Here's the drawing with two shaded views (mm, measured from the low corner). I have some questions. Coordinates: 2 decimals unless noted, no trailing zeros. Write each loop counter-clockwise with the first axis right and the second up, starting at its lowest first coordinate (ties: lowest second). Pieces come first, ordered by that corner, then holes. Notation, with made-up numbers: (68, -28) -> (106, -28) arc R9 cw to (106, -16) -> close; hole circle Ø8 at (62.25, 76). An arc over 180 degrees is marked (long way). Use one line per item in the form item = value.
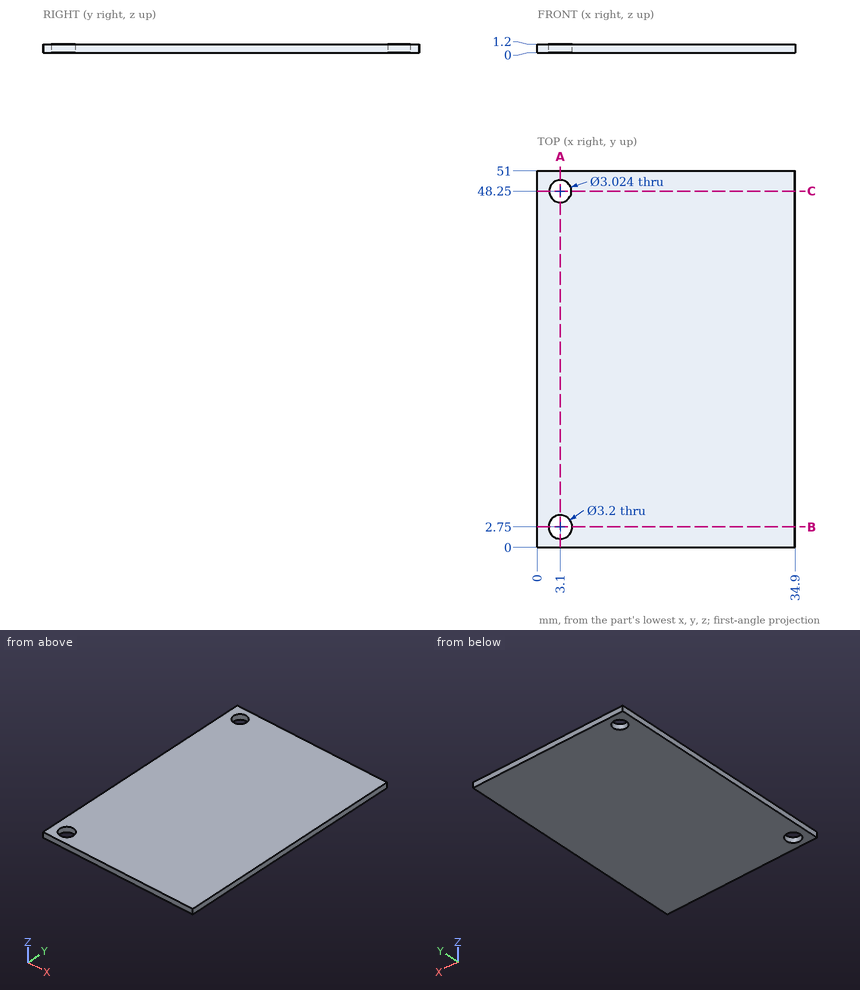
Q1. If I drill on line 1 (Y direction, x = 3.1, z = 0.35); line 2 (Y direction, x = 4, z = 0.5) (1 decimal), over which ranges is the centre line in solid material (lowest first)? Write a range as from..to.
Return value:
line_1 = 0..1.15, 4.35..46.74, 49.76..51
line_2 = 0..1.4, 4.1..47, 49.5..51
Q2. Will this pin go through, and if not, where does the flat tip stop? pin 1 (3 mm diameter, centred on x = 15.5, y = 24, fed in from -Z).
Return value:
pin_1 = 0
Q3. Suppose I cut it at C-C (y = 48.25). Write out the boundary of the cut face in (x, z).
Return value:
outline = (0, 0) -> (1.59, 0) -> (1.59, 1.2) -> (0, 1.2) -> close; (4.61, 0) -> (34.9, 0) -> (34.9, 1.2) -> (4.61, 1.2) -> close
Q4. Suppose I cut it at B-B (y = 2.75). Write out the boundary of the cut face in (x, z).
Return value:
outline = (0, 0) -> (1.5, 0) -> (1.5, 1.2) -> (0, 1.2) -> close; (4.7, 0) -> (34.9, 0) -> (34.9, 1.2) -> (4.7, 1.2) -> close
Q5. Suppose I cut it at A-A (x = 3.1). Write out the boundary of the cut face in (y, z).
Return value:
outline = (0, 0) -> (1.15, 0) -> (1.15, 1.2) -> (0, 1.2) -> close; (4.35, 0) -> (46.74, 0) -> (46.74, 1.2) -> (4.35, 1.2) -> close; (49.76, 0) -> (51, 0) -> (51, 1.2) -> (49.76, 1.2) -> close
